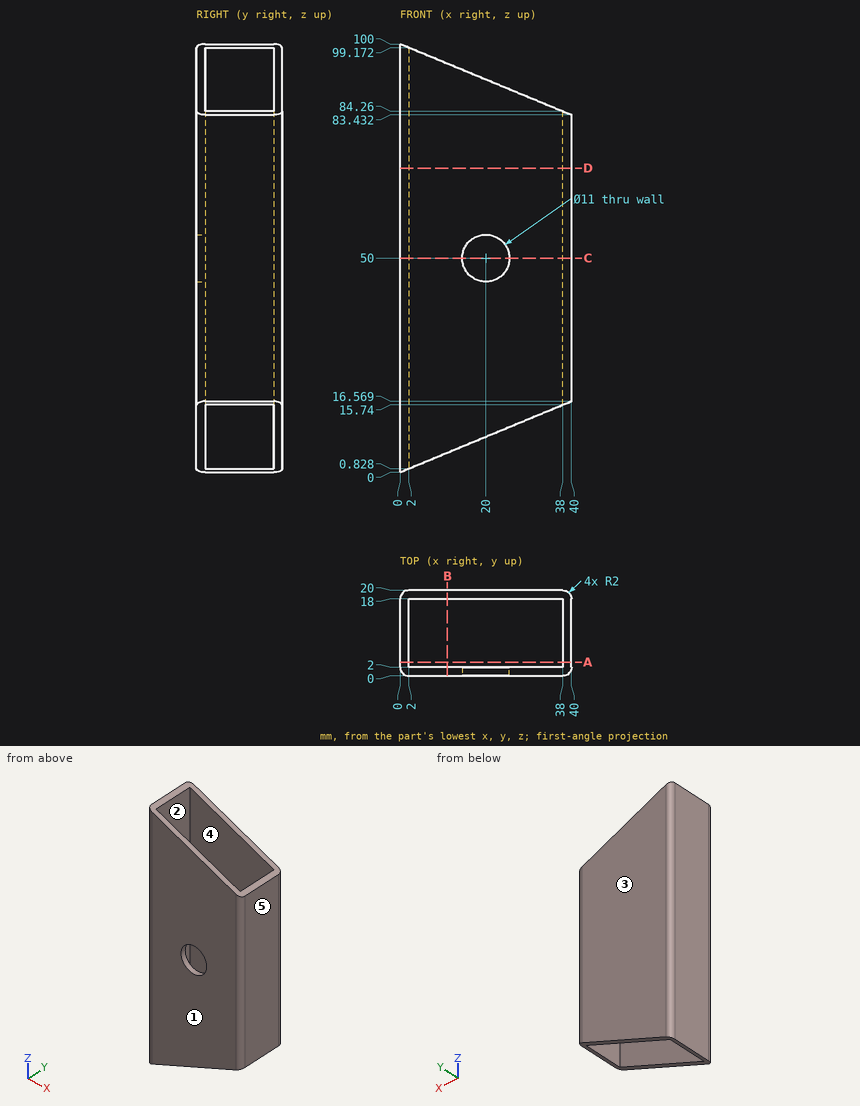
Design review of the part shown in the three views and the two pictorial views. Dimensions are in mm from the part's minimum x, y and z. A direction names the side the tool comes from. Give positions to 0.01 mm unless a question says otherwise; leave off trailing zeros. Write each loop counter-clockwise with the first axis right and the second up, starting at its lowest first coordinate (ties: lowest second). Pieces come first, ordered by that corner, then holes.
Item 1: Take a section at C-C (z = 50). Give the boundary of the cut face in (x, y).
Item 2: The part is to be moulded in two halves that separate along Y. For the marked faces 3, 4 and 5, say which applies: +Y half, -Y half, draft (parallel to the pull), parting line (faces both ways), or undercut.
Item 3: Insertion check: P1, Ø8, axis at x = 22, y = 11.5, coming from the +Z side. The pin has a flat end and moves straight along its axis. Give the tip position at first contact, or say it passes through.
Item 4: Machinability: for the marked faces 1 and 2, which of the approach directions +Z, -Z, +X, -X, +Y, -Y give a long, thin tool a straight path to every point of the face, cutting with its end or side? Answer none if there is none.
Item 5: Take a section at A-A (y = 3.25). Give the boundary of the cut face in (x, z).
Item 6: Take a section at D-D (z = 71). Give the boundary of the cut face in (x, y).
Item 7: Take a section at B-B (x = 11). Give the boundary of the cut face in (y, z).
Item 8: Wall thickness on probe 1 along X at (y, z) = (10.5, 17.5); probe 2 along Y at (x, z) = (8.5, 56.5); probe 3 along Y at (x, z) = (21, 51): over which ranges is each line inside the solid? List them lowest first.
Established:
1. outline: (0, 2) arc R2 ccw to (2, 0) - (14.5, 0) - (14.5, 2) - (2, 2) - (2, 18) - (38, 18) - (38, 2) - (25.5, 2) - (25.5, 0) - (38, 0) arc R2 ccw to (40, 2) - (40, 18) arc R2 ccw to (38, 20) - (2, 20) arc R2 ccw to (0, 18) - close
2. face 3: +Y half
2. face 4: undercut
2. face 5: draft
3. P1: passes through
4. face 1: +Z, -Z, +X, -X, -Y
4. face 2: +Z, -Z
5. outline: (0, 0) - (2, 0.83) - (2, 99.17) - (0, 100) - close; (38, 15.74) - (40, 16.57) - (40, 83.43) - (38, 84.26) - close
6. outline: (0, 2) arc R2 ccw to (2, 0) - (38, 0) arc R2 ccw to (40, 2) - (40, 18) arc R2 ccw to (38, 20) - (2, 20) arc R2 ccw to (0, 18) - close; hole (2, 2) - (38, 2) - (38, 18) - (2, 18) - close
7. outline: (0, 4.56) - (2, 4.56) - (2, 95.44) - (0, 95.44) - close; (18, 4.56) - (20, 4.56) - (20, 95.44) - (18, 95.44) - close
8. probe 1: x = 0 to 2, 38 to 40
8. probe 2: y = 0 to 2, 18 to 20
8. probe 3: y = 18 to 20
